```python
from build123d import *

# Parameters (mm, degrees)
SKETCH1_W           = 596.9
SKETCH1_H           = 17.78
BOSS_EXTRUDE1_DEPTH = 3.175
SKETCH3_W           = 37.846
SKETCH3_H           = 3.175
BOSS_EXTRUDE2_DEPTH = 3.175
SKETCH4_R           = 3.556
SKETCH4_R_2         = 4.8895
CUT_EXTRUDE1_DEPTH  = 299.710641508
CUT_EXTRUDE3_DEPTH  = 299.710641508


with BuildPart() as part:
    # Sketch1 → Boss-Extrude1 (new body)
    with BuildSketch(Plane.XY):
        Rectangle(SKETCH1_W, SKETCH1_H)
    extrude(amount=BOSS_EXTRUDE1_DEPTH)

    # Sketch3 → Boss-Extrude2 (add)
    with BuildSketch(Plane(origin=(0, 8.89, 0), x_dir=(1, 0, 0), z_dir=(0, 1, 0))):
        with Locations((-199.093666667, -1.5875)):
            Rectangle(SKETCH3_W, SKETCH3_H)
        with Locations((-99.610333333, -1.5875)):
            Rectangle(SKETCH3_W, SKETCH3_H)
        with Locations((-0.127, -1.5875)):
            Rectangle(SKETCH3_W, SKETCH3_H)
        with Locations((99.483333333, -1.5875)):
            Rectangle(SKETCH3_W, SKETCH3_H)
        with Locations((198.966666751, -1.5875)):
            Rectangle(SKETCH3_W, SKETCH3_H)
    boss_extrude2 = extrude(amount=BOSS_EXTRUDE2_DEPTH)

    # Mirror1: Boss-Extrude2 across plane
    add(boss_extrude2.mirror(Plane.ZX))

    # Sketch4 → Cut-Extrude1 (cut, through all)
    with BuildSketch(Plane(origin=(0, 0, 0), x_dir=(-1, 0, 0), z_dir=(0, 0, -1))):
        with Locations((-288.925, 0)):
            Circle(SKETCH4_R)
        with Locations((-244.475, 0)):
            Circle(SKETCH4_R)
        with Locations((-266.7, 0)):
            Circle(SKETCH4_R_2)
    cut_extrude1 = extrude(amount=-CUT_EXTRUDE1_DEPTH, mode=Mode.SUBTRACT)

    # Mirror2: Cut-Extrude1 across plane
    add(cut_extrude1.mirror(Plane(origin=(0, 0, 0), x_dir=(0, 0, 1), z_dir=(1, 0, 0))), mode=Mode.SUBTRACT)

    # Sketch6 → Cut-Extrude3 (cut, through all)
    with BuildSketch(Plane.XY.offset(3.175)):
        with BuildLine():
            Line((-208.618666667, 3.81), (-189.568666667, 3.81))
            ThreePointArc((-189.568666667, 3.81), (-185.758666667, 0), (-189.568666667, -3.81))
            Line((-189.568666667, -3.81), (-208.618666667, -3.81))
            ThreePointArc((-208.618666667, -3.81), (-212.428666667, 0), (-208.618666667, 3.81))
        make_face()
        with BuildLine():
            Line((-109.135333333, 3.81), (-90.085333333, 3.81))
            ThreePointArc((-90.085333333, 3.81), (-86.275333333, 0), (-90.085333333, -3.81))
            Line((-90.085333333, -3.81), (-109.135333333, -3.81))
            ThreePointArc((-109.135333333, -3.81), (-112.945333333, 0), (-109.135333333, 3.81))
        make_face()
        with BuildLine():
            Line((-9.652, 3.81), (9.398, 3.81))
            ThreePointArc((9.398, 3.81), (13.208, 0), (9.398, -3.81))
            Line((9.398, -3.81), (-9.652, -3.81))
            ThreePointArc((-9.652, -3.81), (-13.462, 0), (-9.652, 3.81))
        make_face()
        with BuildLine():
            Line((89.831333333, 3.81), (108.881333333, 3.81))
            ThreePointArc((108.881333333, 3.81), (112.691333333, 0), (108.881333333, -3.81))
            Line((108.881333333, -3.81), (89.831333333, -3.81))
            ThreePointArc((89.831333333, -3.81), (86.021333333, 0), (89.831333333, 3.81))
        make_face()
        with BuildLine():
            Line((189.314666667, 3.81), (208.364666667, 3.81))
            ThreePointArc((208.364666667, 3.81), (212.174666667, 0), (208.364666667, -3.81))
            Line((208.364666667, -3.81), (189.314666667, -3.81))
            ThreePointArc((189.314666667, -3.81), (185.504666667, 0), (189.314666667, 3.81))
        make_face()
        with BuildLine():
            Line((-158.877, 3.81), (-139.827, 3.81))
            ThreePointArc((-139.827, 3.81), (-136.017, 0), (-139.827, -3.81))
            Line((-139.827, -3.81), (-158.877, -3.81))
            ThreePointArc((-158.877, -3.81), (-162.687, 0), (-158.877, 3.81))
        make_face()
        with BuildLine():
            Line((-59.319456458, 3.81), (-40.417876875, 3.81))
            ThreePointArc((-40.417876875, 3.81), (-36.607876875, 0), (-40.417876875, -3.81))
            Line((-40.417876875, -3.81), (-59.319456458, -3.81))
            ThreePointArc((-59.319456458, -3.81), (-63.129456458, 0), (-59.319456458, 3.81))
        make_face()
        with BuildLine():
            Line((40.089666667, 3.81), (59.139666667, 3.81))
            ThreePointArc((59.139666667, 3.81), (62.949666667, 0), (59.139666667, -3.81))
            Line((59.139666667, -3.81), (40.089666667, -3.81))
            ThreePointArc((40.089666667, -3.81), (36.279666667, 0), (40.089666667, 3.81))
        make_face()
        with BuildLine():
            Line((139.573, 3.81), (158.623, 3.81))
            ThreePointArc((158.623, 3.81), (162.433, 0), (158.623, -3.81))
            Line((158.623, -3.81), (139.573, -3.81))
            ThreePointArc((139.573, -3.81), (135.763, 0), (139.573, 3.81))
        make_face()
    extrude(amount=-CUT_EXTRUDE3_DEPTH, mode=Mode.SUBTRACT)


solid = part.part
```
Source: CAD feature listing. Evaluate the final solid. Frame: model axes, mm. Give positions to 0.01 mm unless a question says otherwise; leave off trailing zeros. Loops run counter-clockwise (first coordinate to the right, second up) from the corner with the lowest first, then second, coordinate; pieces in that order, holes last. Notation, with made-up numbers: (-39, 38.25) -> (16, 38.25) arc R27 ccw to (16, 61.25) -> close; hole circle Ø7 at (29.25, -12). An arc over 180 degrees is marked (long way). Put each result on its own line as item: value. Start each with the question number.
1) Cut plane C-C (x = 169). Return loops of the section in (y, z) (3 decimals), then the cut area to 3 significant figures.
2) Draft query along Y for faces 1 (the face through (-4, -5, 3.175)), 2 (the face through (-271.585, 0.215, 1.565)). Return one class per face: released by +Y, released by -Y, zero draft, split by the parting line, or undercut.
3) Contact query for flat-ended pins moving along their axis: P1, Ø1.6, axis at y = 11, z = 1, coming from the +X side; P2, Ø8, axis at x = 140, y = -2, coming from the -Z side; P3, Ø1, axis at x = -154, z = 1, coming from the +Y side; P4, Ø1.6, axis at x = -148.5, z = 1, coming from the -Y side. Output: stop coordinate, or through.
4) Cut plane A-A (x = -266.7). Return loops of the section in (y, z) (1 decimal).
5) Cut plane B-B (z = 2.1). State how many separate pieces and enclosed holes the cut face has, then the cut area to 3 significant figures.
6) Material intervals for probe 1 along X at (y, z) = (10.75, 2.3); probe 2 along Y at (x, z) = (-266.7, 1.1); probe 3 along Y at (x, z) = (-3, 0.95) (3 decimals), sorted ascending.
Results are:
1. outline: (-8.89, 0) -> (8.89, 0) -> (8.89, 3.175) -> (-8.89, 3.175) -> close
1. area: 56.5 mm2
2. face 1: zero draft
2. face 2: undercut
3. P1: stops at x = 217.89
3. P2: stops at z = 0
3. P3: stops at y = 8.89
3. P4: stops at y = -8.89
4. outline: (-8.9, 0) -> (-4.9, 0) -> (-4.9, 3.2) -> (-8.9, 3.2) -> close; (4.9, 0) -> (8.9, 0) -> (8.9, 3.2) -> (4.9, 3.2) -> close
5. separate pieces: 1
5. enclosed holes: 15
5. area: 9,790 mm2
6. probe 1: x = -218.02 to -180.17, -118.53 to -80.69, -19.05 to 18.8, 80.56 to 118.41, 180.04 to 217.89
6. probe 2: y = -8.89 to -4.89, 4.89 to 8.89
6. probe 3: y = -12.065 to -3.81, 3.81 to 12.065
